Design review of the part built by this model. Coordinates are the model's own, in mm. A direction names the side the tool comes from. Coordinates: 2 decimals unless noted, no trailing zeros. Loops run counter-clockwise (first coordinate to the right, second up) from the corner with the lowest first, then second, coordinate; pieces in that order, holes last. Notation, with made-up numbers: (-28.5, 10) - (8.5, 10) arc R16 cw to (8.5, 30) - close; hole circle Ø10 at (20, -35.5). An arc over 180 degrees is marked (long way). Return JSON: item names as keys, results as strings. Group by question number.
from build123d import *

# Parameters (mm, degrees)
CROQUIS1_W              = 180
CROQUIS1_H              = 180
CROQUIS1_R              = 2.5
CROQUIS1_W_2            = 158
CROQUIS1_H_2            = 158
SALIENTE_EXTRUIR1_DEPTH = 4
CROQUIS2_W              = 5.5
CROQUIS2_H              = 63
CROQUIS2_W_2            = 63
CROQUIS2_H_2            = 5.5
SALIENTE_EXTRUIR2_DEPTH = 4


with BuildPart() as part:
    # Croquis1 → Saliente-Extruir1 (new body)
    with BuildSketch(Plane(origin=(0, 0, 0), x_dir=(1, 0, 0), z_dir=(0, 1, 0))):
        with Locations((90, 90)):
            Rectangle(CROQUIS1_W, CROQUIS1_H)
        with Locations(Location((5, 175, 0), (0, 0, 270))):
            Circle(CROQUIS1_R, mode=Mode.SUBTRACT)
        with Locations(Location((175, 175, 0), (0, 0, 270))):
            Circle(CROQUIS1_R, mode=Mode.SUBTRACT)
        with Locations(Location((175, 5, 0), (0, 0, 270))):
            Circle(CROQUIS1_R, mode=Mode.SUBTRACT)
        with Locations(Location((5, 5, 0), (0, 0, 270))):
            Circle(CROQUIS1_R, mode=Mode.SUBTRACT)
        with Locations((90, 90)):
            Rectangle(CROQUIS1_W_2, CROQUIS1_H_2, mode=Mode.SUBTRACT)
    extrude(amount=SALIENTE_EXTRUIR1_DEPTH)

    # Croquis2 → Saliente-Extruir2 (add)
    with BuildSketch(Plane(origin=(0, 4, 0), x_dir=(1, 0, 0), z_dir=(0, 1, 0))):
        with Locations((2.75, 137)):
            Rectangle(CROQUIS2_W, CROQUIS2_H)
        with Locations((43, 177.25)):
            Rectangle(CROQUIS2_W_2, CROQUIS2_H_2)
        with Locations((137, 177.25)):
            Rectangle(CROQUIS2_W_2, CROQUIS2_H_2)
        with Locations((177.25, 137)):
            Rectangle(CROQUIS2_W, CROQUIS2_H)
        with Locations((177.25, 43)):
            Rectangle(CROQUIS2_W, CROQUIS2_H)
        with Locations((137, 2.75)):
            Rectangle(CROQUIS2_W_2, CROQUIS2_H_2)
        with Locations((43, 2.75)):
            Rectangle(CROQUIS2_W_2, CROQUIS2_H_2)
        with Locations((2.75, 43)):
            Rectangle(CROQUIS2_W, CROQUIS2_H)
    extrude(amount=SALIENTE_EXTRUIR2_DEPTH)


solid = part.part
Item 1: Draft analysis for pull direction X (two halves, no side actions). For faces 6 (the face through (74.5, 6, -177)), 7 (the face through (0, 3, -89)), 8 (the face through (43, 8, -3)), 9 (the face through (89, 2, -169)), state which applies: pulls with the +X half, pulls with the -X half, needs draft (parallel to the pull), parting line crosses it, or undercut.
Item 2: Add section B-B (y = 1.5). State the section outline as (x, z) points.
Item 3: Add section C-C (z = -137). State the section outline as (x, y) points, then the cut area to 3 significant figures.
Item 4: To check wall thickness, follow line 1 (X direction, y = 2.85, z = -175); line 2 (Z direction, x = 121, y = 6); line 3 (Z direction, x = 175, y = 2.5). State the ranges of each line that lie inside material, in increasing order. Write a range as from..to.
Item 5: For P1, Ø2, axis at y = 5.5, z = -1.5, coming from the +X side; P2, Ø1.2, axis at x = 177, y = 5.5, coming from the +Z side; P3, Ø3, axis at y = 6, z = -3.5, coming from the -X side; P4, Ø4.5, axis at x = 4, y = 5, coming from the -Z side, all flat-tipped, find the tip position at first contact; note any pin that passes through.
Item 6: Add section A-A (x = 28). State the section outline as (y, z) points.
Item 7: For faces 1 (the face through (3, 6, -11.5)), 2 (the face through (168.5, 6, -3)), 3 (the face through (89, 2, -11)), 4 (the face through (3, 6, -105.5)), 5 (the face through (105.5, 6, -177)), list the 3-axis set-ups (+Z, -Z, +X, -X, +Y, -Y) from which the entire face can be reached by the end or side of a thin tool; tool diameter is ignored.
Answers below:
{
 "1": {"face 6": "undercut", "face 7": "pulls with the -X half", "face 8": "needs draft", "face 9": "undercut"},
 "2": {"outline": "(0, -180) - (180, -180) - (180, 0) - (0, 0) - close; hole circle Ø5 at (5, -175); hole circle Ø5 at (5, -5); hole (11, -169) - (169, -169) - (169, -11) - (11, -11) - close; hole circle Ø5 at (175, -175); hole circle Ø5 at (175, -5)"},
 "3": {"outline": "(0, 0) - (11, 0) - (11, 4) - (5.5, 4) - (5.5, 8) - (0, 8) - close; (169, 0) - (180, 0) - (180, 8) - (174.5, 8) - (174.5, 4) - (169, 4) - close", "area": "132 mm^2"},
 "4": {"line 1": "x = 0..2.5, 7.5..172.5, 177.5..180", "line 2": "z = -180..-174.5, -5.5..0", "line 3": "z = -180..-177.5, -172.5..-7.5, -2.5..0"},
 "5": {"P1": "stops at x = 168.5", "P2": "stops at z = -11.5", "P3": "stops at x = 11.5", "P4": "stops at z = -180"},
 "6": {"outline": "(0, -180) - (8, -180) - (8, -174.5) - (4, -174.5) - (4, -169) - (0, -169) - close; (0, -11) - (4, -11) - (4, -5.5) - (8, -5.5) - (8, 0) - (0, 0) - close"},
 "7": {"face 1": "+Z, +X, -X, +Y", "face 2": "+Z, -Z, +X, +Y", "face 3": "+Y, -Y", "face 4": "+X, -X, +Y", "face 5": "+Z, -Z, +Y"}
}
